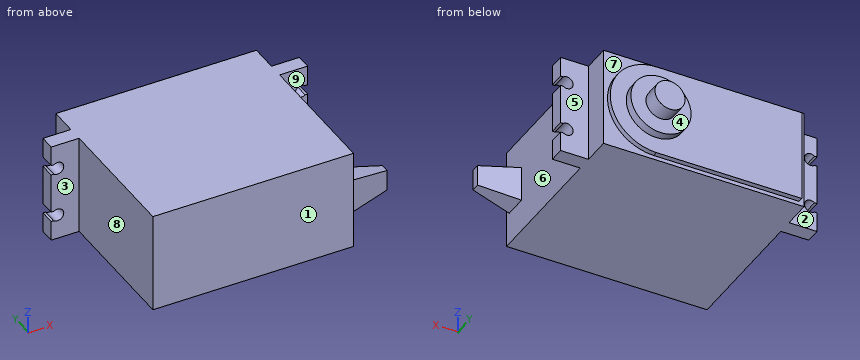
```python
from build123d import *

# Parameters (mm, degrees)
RESSALTO_EXTRUS_O1_DEPTH = 10
CORTE_EXTRUS_O1_DEPTH    = 10
RESSALTO_EXTRUS_O2_DEPTH = 1
ESBO_O4_R                = 3
RESSALTO_EXTRUS_O3_DEPTH = 5
ESBO_O5_R                = 6
RESSALTO_EXTRUS_O4_DEPTH = 1.7
ESBO_O7_W                = 7
ESBO_O7_H                = 4.5
RESSALTO_EXTRUS_O5_DEPTH = 8
RESSALTO_EXTRUS_O5_TAPER = 10


with BuildPart() as part:
    # Esboço1 → Ressalto-extrusão1 (new, symmetric)
    with BuildSketch(Plane.XY):
        Polygon((20, -0.767915455), (25.568877633, -0.767915455), (25.568877633, -3.767915455), (20, -3.767915455), (20, -30.767915455), (-20, -30.767915455), (-20, -3.767915455), (-25.568877633, -3.767915455), (-25.568877633, -0.767915455), (-20, -0.767915455), (-20, 4.732084545), (20, 4.732084545), align=None)
    extrude(amount=RESSALTO_EXTRUS_O1_DEPTH, both=True)

    # Esboço6 → Corte-extrusão1 (cut)
    with BuildSketch(Plane(origin=(0, -0.767915455, 0), x_dir=(1, 0, 0), z_dir=(0, 1, 0))):
        with BuildLine():
            Line((25.071445053, 4), (25.568877633, 4))
            Line((25.568877633, 4), (25.568877633, 6))
            Line((25.568877633, 6), (25.071445053, 6))
            ThreePointArc((25.071445053, 6), (23.061122367, 5), (25.071445053, 4))
        make_face()
        with BuildLine():
            Line((25.568877633, -6), (25.568877633, -4))
            Line((25.568877633, -4), (25.071445053, -4))
            ThreePointArc((25.071445053, -4), (23.061122367, -5), (25.071445053, -6))
            Line((25.071445053, -6), (25.568877633, -6))
        make_face()
        with BuildLine():
            ThreePointArc((-25.071445053, 6), (-23.061122367, 5), (-25.071445053, 4))
            Line((-25.071445053, 4), (-25.568877633, 4))
            Line((-25.568877633, 4), (-25.568877633, 6))
            Line((-25.568877633, 6), (-25.071445053, 6))
        make_face()
        with BuildLine():
            ThreePointArc((-25.071445053, -4), (-23.061122367, -5), (-25.071445053, -6))
            Line((-25.071445053, -6), (-25.568877633, -6))
            Line((-25.568877633, -6), (-25.568877633, -4))
            Line((-25.568877633, -4), (-25.071445053, -4))
        make_face()
    extrude(amount=-CORTE_EXTRUS_O1_DEPTH, mode=Mode.SUBTRACT)

    # Esboço3 → Ressalto-extrusão2 (add)
    with BuildSketch(Plane(origin=(0, 4.732084545, 0), x_dir=(1, 0, 0), z_dir=(0, 1, 0))):
        with BuildLine():
            Line((-19, 9.202511885), (10.015, 9.202511885))
            ThreePointArc((10.015, 9.202511885), (19.216883893, -0.107507336), (9.8, -9.2))
            Line((9.8, -9.2), (-19, -9.2))
            Line((-19, -9.2), (-19, 9.202511885))
        make_face()
    extrude(amount=RESSALTO_EXTRUS_O2_DEPTH)

    # Esboço4 → Ressalto-extrusão3 (add)
    with BuildSketch(Plane(origin=(0, 5.732084545, 0), x_dir=(1, 0, 0), z_dir=(0, 1, 0))):
        with Locations(Location((10.015, 0, 0), (0, 0, 180))):
            Circle(ESBO_O4_R)
    extrude(amount=RESSALTO_EXTRUS_O3_DEPTH)

    # Esboço5 → Ressalto-extrusão4 (add)
    with BuildSketch(Plane(origin=(0, 5.732084545, 0), x_dir=(1, 0, 0), z_dir=(0, 1, 0))):
        with Locations(Location((10.015, 0, 0), (0, 0, 180))):
            Circle(ESBO_O5_R)
    extrude(amount=RESSALTO_EXTRUS_O4_DEPTH)

    # Esboço7 → Ressalto-extrusão5 (add)
    with BuildSketch(Plane(origin=(20, 0, 0), x_dir=(0, 0, -1), z_dir=(1, 0, 0))):
        with Locations((0, -27.517915455)):
            Rectangle(ESBO_O7_W, ESBO_O7_H)
    extrude(amount=RESSALTO_EXTRUS_O5_DEPTH, taper=RESSALTO_EXTRUS_O5_TAPER)


solid = part.part
```
Geometry check sheet. Reference: the model listing, model coordinates, mm. Face numbers are marked on the shaded views. A direction names the side the tool comes from. Coordinates: 2 decimals unless noted, no trailing zeros. Order: outer loops, then holes, each group sorted by start corner. A loop starts at its lowest first (then second) coordinate and runs counter-clockwise, first axis right, second up.
Item 1: Depth check by flat-ended pin: pin 1 (2.5 mm diameter, centred on y = -2, z = -0.5, fed in from +X); pin 2 (9 mm diameter, centred on x = 0.5, z = -3, fed in from +Y); pin 3 (4 mm diameter, centred on x = -24.315, z = 5, fed in from -Y). Enter the tip coordinate at first touch or a pass-through.
Item 2: Tool access check on the marked faces 1, 2, 3, 4 and 5. Record the directions out of +Z, -Z, +X, -X, +Y, -Y that give a thin tool (end or side, any length) a straight path to the whole face; none if there is none.
Item 3: Section check B-B (z = -5). Enter the section's corners in (x, y), plus the area to 3 significant figures.
Item 4: Section check C-C (y = -18). Enter the section's corners in (x, z).
Item 5: Mould release check, pull along Y, two halves, no side actions. Record for the marked faces 6, 7, 8 and 9: released by +Y, released by -Y, zero draft, split by the parting line, or undercut.
Item 6: Section check D-D (x = 5.5). Enter the section's corners in (y, z).
Item 7: Scan lines: line 1 along Y through (x, z) = (-8, 1.25); line 2 along X through (y, z) = (-9, 8.5); line 3 along Y through (x, z) = (20.5, -3.25). Record each from-to range of solid material in increasing order.
Item 8: Section check A-A (x = -17.5). Enter the section's corners in (y, z).
Check sheet entries:
1. pin 1: stops at x = 25.57
1. pin 2: stops at y = 7.43
1. pin 3: stops at y = -3.77
2. face 1: +Z, -Z, +X, -X, -Y
2. face 2: +Z, -Z, -X, +Y
2. face 3: +Z, -Z, -X, -Y
2. face 4: +Y
2. face 5: +Z, -Z, +X, +Y
3. outline: (-23.06, -3.77) - (-20, -3.77) - (-20, -30.77) - (20, -30.77) - (20, -3.77) - (23.06, -3.77) - (23.06, -0.77) - (20, -0.77) - (20, 4.73) - (17.74, 4.73) - (17.74, 5.73) - (13.33, 5.73) - (13.33, 7.43) - (6.7, 7.43) - (6.7, 5.73) - (-19, 5.73) - (-19, 4.73) - (-20, 4.73) - (-20, -0.77) - (-23.06, -0.77) - close
3. area: 1,490 mm2
4. outline: (-20, -10) - (20, -10) - (20, 10) - (-20, 10) - close
5. face 6: undercut
5. face 7: released by +Y
5. face 8: zero draft
5. face 9: undercut
6. outline: (-30.77, -10) - (4.73, -10) - (4.73, -9.2) - (5.73, -9.2) - (5.73, -3.95) - (7.43, -3.95) - (7.43, 3.95) - (5.73, 3.95) - (5.73, 9.2) - (4.73, 9.2) - (4.73, 10) - (-30.77, 10) - close
7. line 1: y = -30.77 to 5.73
7. line 2: x = -20 to 20
7. line 3: y = -29.68 to -25.36, -3.77 to -0.77
8. outline: (-30.77, -10) - (4.73, -10) - (4.73, -9.2) - (5.73, -9.2) - (5.73, 9.2) - (4.73, 9.2) - (4.73, 10) - (-30.77, 10) - close
